The listing builds one solid part. Answer for the finished solid, in the listing's coordinates (mm). A direction names the side the tool comes from. Round coordinates to 2 decimals unless told otherwise and drop trailing zeros. Loops run counter-clockwise (first coordinate to the right, second up) from the corner with the lowest first, then second, coordinate; pieces in that order, holes last. Notation, with made-up numbers: M -13,52.5 L 9,52.5 A16 ccw 9,80.5 Z; hole C 11.5,15 d6. An arc over 180 degrees is marked long. Put each result on its own line as item: value. Start each with the question number.
(1) Section A-A, the plane y = 0 is taken. Determine the outline of the cut face in (x, z), then the cut area to 3 significant figures.
(2) Straight lines are drawn through the part: line 1 (X direction, y = 0, z = -13.5); line 2 (Y direction, x = 0, z = 21.5); line 3 (Y direction, x = -13.5, z = 29). For each, find the intervals that lie inside material, in ascending order.
(3) Section B-B, the plane x = 16 is taken. Determine the outline of the cut face in (y, z), then the cut area to 3 significant figures.
(4) Section C-C, the plane z = 14.5 is taken. Determine the outline of the cut face in (x, y).
(5) Determine the mould class of faces 4 (the face through (-9, 25, 45)), 5 (the face through (1.284, 29.973, 0.63)), 6 (the face through (2.5, -28, 27)) for opening direction X: released by +X, released by -X, zero draft, split by the parting line, or undercut.
(6) Which of the six approach directions +Z, -Z, +X, -X, +Y, -Y give full straight-line access (tool end or side, diameter ignored) to faces 1 (the face through (-10.75, -26.74, 0.2)), 2 (the face through (-2.5, -28, -28)), 3 (the face through (-9, 25, -45))?
(7) Section D-D, the plane x = 0 is taken. Determine the outline of the cut face in (y, z), then the cut area to 3 significant figures.
(8) Flat-ended cylindrical pins translate along their axes: P1, Ø3, axis at y = 19, z = -12.5, coming from the +X side; P2, Ø4.5, axis at y = -28, z = -27, coming from the +X side; P3, Ø6, axis at y = 10.5, z = 9.5, coming from the +X side. Find the tip coordinate at first contact, or state that the pin passes through.
```python
from build123d import *

# Parameters (mm, degrees)
SKETCH009_R       = 30
SKETCH009_R_2     = 26
PAD002_DEPTH      = 45
PAD002_DEPTH_BACK = 45
SKETCH010_R       = 10.75
POCKET007_DEPTH   = 30.001
SKETCH027_W       = 5
SKETCH027_H       = 90
POCKET012_DEPTH   = 30.001


with BuildPart() as part:
    # Sketch009 → Pad002 (new body, two sides)
    with BuildSketch(Plane.XY) as pad002_sk:
        Circle(SKETCH009_R)
        Circle(SKETCH009_R_2, mode=Mode.SUBTRACT)
    extrude(amount=PAD002_DEPTH)
    extrude(pad002_sk.sketch, amount=-PAD002_DEPTH_BACK)

    # Sketch010 → Pocket007 (cut, through all)
    with BuildSketch(Plane.XZ):
        Circle(SKETCH010_R)
    extrude(amount=POCKET007_DEPTH, mode=Mode.SUBTRACT)

    # Sketch027 → Pocket012 (cut, through all)
    with BuildSketch(Plane.XZ):
        Rectangle(SKETCH027_W, SKETCH027_H)
    extrude(amount=POCKET012_DEPTH, mode=Mode.SUBTRACT)


solid = part.part
```
Recorded:
1. outline: M -30,-45 L -26,-45 L -26,45 L -30,45 Z; M 26,-45 L 30,-45 L 30,45 L 26,45 Z
1. area: 720 mm²
2. line 1: x = -30 to -26, 26 to 30
2. line 2: y = 26 to 30
2. line 3: y = -26.79 to -22.22, 22.22 to 26.79
3. outline: M -25.38,-45 L -20.49,-45 L -20.49,45 L -25.38,45 Z; M 20.49,-45 L 25.38,-45 L 25.38,45 L 20.49,45 Z
3. area: 879 mm²
4. outline: M -2.5,-29.9 L -2.5,-25.88 A26 cw long 2.5,-25.88 L 2.5,-29.9 A30 ccw long Z
5. face 4: zero draft
5. face 5: split by the parting line
5. face 6: undercut
6. face 1: -Y
6. face 2: +Z, -Z, -Y
6. face 3: -Z, +X, -X, +Y, -Y
7. outline: M 26,-45 L 30,-45 L 30,45 L 26,45 Z
7. area: 360 mm²
8. P1: stops at x = 24.37
8. P2: stops at x = 15.39
8. P3: stops at x = 29.05
